Design review of the part built by this model. Coordinates are the model's own, in mm. Face numbers are marked on the shaded views. A direction names the side the tool comes from. Coordinates: 2 decimals unless noted, no trailing zeros. Loops run counter-clockwise (first coordinate to the right, second up) from the corner with the lowest first, then second, coordinate; pieces in that order, holes last. Notation, with made-up numbers: (25.25, 26.25) -> (75.25, 26.25) arc R31 ccw to (75.25, 58.25) -> close; hole circle Ø4 at (-8, 86). An arc over 180 degrees is marked (long way). Use CSV: the item, a comma, the result in double quotes.
Autodesk Inventor part; units mm, degrees
ref_plane "YZ Plane" through (0, 0, 0) normal (1, 0, 0) x (0, 1, 0)
ref_plane "XZ Plane" through (0, 0, 0) normal (0, 1, 0) x (-1, 0, 0)
ref_plane "XY Plane" through (0, 0, 0) normal (0, 0, 1) x (1, 0, 0)
sketch "Sketch1" plane through (0, 0, 0) normal (0, 0, 1) x (1, 0, 0)
  line L0 (0, 0) -> (38, 0) construction
  arc A0 (62.7487, -10.2513) -> (38, 0) centre (38, -35) ccw construction
  arc A1 (62.7487, -10.2513) -> (76.8909, -10.2513) centre (69.8198, -3.1802) ccw construction
  arc A2 (80, -8.9625) -> (76.8909, -10.2513) centre (80.0021, -13.3625) ccw construction
  line L1 (38, 0) -> (38, -35) construction
  line L2 (38, -35) -> (69.8198, -3.1802) construction
  line L3 (69.8198, -3.1802) -> (80.0021, -13.3625) construction
  line L4 (5.4544, 2.5) -> (38, 2.5)
  arc A3 (64.5165, -8.4835) -> (38, 2.5) centre (38, -35) ccw
  arc A4 (64.5165, -8.4835) -> (75.1231, -8.4835) centre (69.8198, -3.1802) ccw
  arc A5 (79.9988, -6.4625) -> (75.1231, -8.4835) centre (80.0021, -13.3625) ccw
  arc A6 (60.981, -12.019) -> (38, -2.5) centre (38, -35) ccw
  arc A7 (60.981, -12.019) -> (78.6586, -12.019) centre (69.8198, -3.1802) ccw
  arc A8 (79.9988, -11.4625) -> (78.6586, -12.019) centre (80.0021, -13.3625) ccw
  line L5 (79.9988, -6.4625) -> (79.9988, -11.4625)
  arc A9 (5.4544, 2.5) -> (5.4544, -2.5) centre (0, 0) ccw
  circle A10 centre (0, 0) radius 3
  line L6 (5.4544, -2.5) -> (38, -2.5)
  dimension "d0" = 38
  dimension "d1" = 35
  dimension "d2" = 10
  dimension "d3" = 4.4
  dimension "d4" = 45
  dimension "d5" = 80
  dimension "d6" = 2.5
  dimension "d8" = 12
  dimension "d9" = 6
extrude "Extrusion1" add sketch "Sketch1" along normal mid plane 70
fillet "Fillet1" radius 3 2 edges at (79.9988, -8.9625, 35) (79.9988, -8.9625, -35)
sketch "Sketch2" plane through (0, 0, 0) normal (0, 1, 0) x (-1, 0, 0)
  line L0 (6, -35) -> (6, 35)
  line L1 (-79.9988, -32) -> (-79.9988, 32)
  line L2 (23.2007, 0) -> (-97.2041, 0) construction
  line L3 (6, 35) -> (-5.4544, 35) construction
  line L4 (6, 35) -> (-17, 35)
  arc A0 (-17, 35) -> (-37.4698, 28.3899) centre (-17, 0) ccw
  arc A1 (-66.9147, 20) -> (-37.4698, 28.3899) centre (-63.7881, 64.8913) ccw
  line L5 (-66.9147, 20) -> (-79.9988, 20)
  line L6 (6, -35) -> (-17, -35)
  arc A2 (-37.4698, -28.3899) -> (-17, -35) centre (-17, 0) ccw
  arc A3 (-37.4698, -28.3899) -> (-66.9147, -20) centre (-63.7881, -64.8913) ccw
  line L7 (-66.9147, -20) -> (-79.9988, -20)
  line L8 (-79.9988, -20) -> (-79.9988, 20) construction
  line L9 (-79.9988, -20) -> (-79.9988, 20)
  line L10 (6, -35) -> (6, -15)
  line L11 (6, -15) -> (-9, -15)
  line L12 (-9, -15) -> (-9, 15)
  line L13 (-9, 15) -> (6, 15)
  line L14 (6, 15) -> (6, 35)
  arc A4 (-39.7468, -7) -> (-39.7468, 7) centre (-30, 0) ccw
  arc A5 (-49, 7) -> (-49, -7) centre (-49, 0) ccw
  line L15 (-49, -7) -> (-39.7468, -7)
  line L16 (-49, 7) -> (-39.7468, 7)
  point P0 (0, 0)
  point P1 (6, 0)
  point P2 (-9, 0)
  dimension "d13" = 17
  dimension "d14" = 35
  dimension "d15" = 40
  dimension "d16" = 45
  dimension "d17" = 30
  dimension "d18" = 15
  dimension "d19" = 12
  dimension "d20" = 7
  dimension "d21" = 30
  dimension "d22" = 19
extrude "Extrusion2" cut sketch "Sketch2" along normal mid plane 70 contours L6 A2 A3 L7 L1 L5 A1 A0 L4 L0 L13 L12 L11 keep common part
properties part number "Part017. Tilting clamo" material "Steel, Carbon"
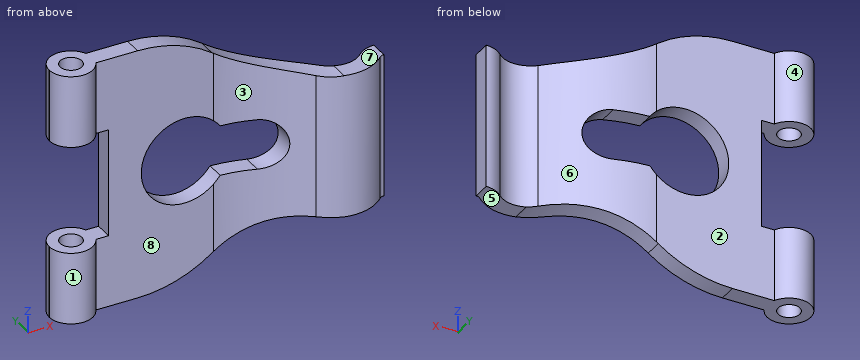
Item 1: Add section B-B (x = 0). Give the boundary of the cut face in (y, z), then the cut area to 3 significant figures.
Checked values:
outline,"(-6, -35) -> (-3, -35) -> (-3, -15) -> (-6, -15) -> close; (-6, 15) -> (-3, 15) -> (-3, 35) -> (-6, 35) -> close; (3, -35) -> (6, -35) -> (6, -15) -> (3, -15) -> close; (3, 15) -> (6, 15) -> (6, 35) -> (3, 35) -> close"
area,"240 mm^2"
Item 2: Add section A-A (z = 17). Give the boundary of the cut face in (x, y).
Checked values:
outline,"(-6, -0.02) arc R6 ccw to (5.45, -2.5) -> (38, -2.5) arc R32.5 cw to (60.98, -12.02) arc R12.5 ccw to (78.66, -12.02) arc R1.9 cw to (80, -11.46) -> (80, -6.46) arc R6.9 ccw to (75.12, -8.48) arc R7.5 cw to (64.52, -8.48) arc R37.5 ccw to (38, 2.5) -> (5.45, 2.5) arc R6 ccw to (-6, 0.02) -> close; hole circle Ø6 at (0, 0)"
Item 3: Clearance check with flat-ended pins moving along their axes: pin 1 (10 mm diameter, centred on x = 76.5, y = -10, fed in from +Z); pin 2 (4 mm diameter, centred on y = -1, z = 4.5, fed in from -X); pin 3 (1.5 mm diameter, centred on x = 10.5, z = 23.5, fed in from +Y). State where each tip first meets the part, or that it passes through.
Checked values:
pin 1,"z = 20"
pin 2,"x = 9"
pin 3,"y = 2.5"
Item 4: Draft analysis for pull direction X (two halves, no side actions). For the marked faces 1, 2, 3 and 4, state which applies: pulls with the +X half, pulls with the -X half, needs draft (parallel to the pull), parting line crosses it, or undercut.
Checked values:
face 1,"undercut"
face 2,"needs draft"
face 3,"undercut"
face 4,"parting line crosses it"
Item 5: Add section D-D (z = 2.5). Give the boundary of the cut face in (x, y).
Checked values:
outline,"(9, -2.5) -> (18.26, -2.5) -> (18.26, 2.5) -> (9, 2.5) -> close; (55.54, -7.64) arc R32.5 cw to (60.98, -12.02) arc R12.5 ccw to (78.66, -12.02) arc R1.9 cw to (80, -11.46) -> (80, -6.46) arc R6.9 ccw to (75.12, -8.48) arc R7.5 cw to (64.52, -8.48) arc R37.5 ccw to (55.54, -1.85) -> close"
Item 6: To check wall thickness, follow line 1 along Y through (x, z) = (0, 27); line 2 along Y through (x, z) = (49, -20); line 3 along Y through (x, z) = (26, 19). State the ranges of each line that lie inside material, in increasing order.
Checked values:
line 1,"-6 to -3, 3 to 6"
line 2,"-4.42 to 0.85"
line 3,"-2.5 to 2.5"
Item 7: Add section C-C (x = 52). Give the boundary of the cut face in (y, z), then the cut area to 3 significant figures.
Checked values:
outline,"(-5.67, -21.46) -> (-0.21, -21.46) -> (-0.21, -6.32) -> (-5.67, -6.32) -> close; (-5.67, 6.32) -> (-0.21, 6.32) -> (-0.21, 21.46) -> (-5.67, 21.46) -> close"
area,"165 mm^2"
Item 8: Machinability: for the marked faces 5, 6, 7 and 8, which of the approach directions +Z, -Z, +X, -X, +Y, -Y give a long, thin tool a straight path to every point of the face, cutting with its end or side? Answer none if there is none.
Checked values:
face 5,"-Z, +X, +Y, -Y"
face 6,"+Z, -Z, +Y"
face 7,"+Z, +X, +Y, -Y"
face 8,"+Z, -Z, -Y"
